```python
from build123d import *

# Parameters (mm, degrees)
BOSS_EXTRUDE1_DEPTH = 50
SKETCH2_W           = 15.285287044
SKETCH2_H           = 2
BOSS_EXTRUDE2_DEPTH = 10
FILLET1_R           = 2
SKETCH3_W           = 10
SKETCH3_H           = 26
SKETCH3_W_2         = 9.897545425
SKETCH3_H_2         = 19
CUT_EXTRUDE1_DEPTH  = 6
SKETCH4_W           = 2
SKETCH4_H           = 5
CUT_EXTRUDE2_DEPTH  = 31
FILLET2_R           = 4
FILLET3_R           = 2


with BuildPart() as part:
    # Sketch1 → Boss-Extrude1 (new body)
    with BuildSketch(Plane(origin=(0, 0, 0), x_dir=(1, 0, 0), z_dir=(0, 1, 0))):
        with BuildLine():
            Line((-5.276963181, 0), (34.723036819, 0))
            Line((34.723036819, 0), (34.723036819, 5))
            Line((34.723036819, 5), (24.723036819, 5))
            Line((24.723036819, 5), (24.723036819, 24))
            Line((24.723036819, 24), (22.365680341, 24))
            ThreePointArc((22.365680341, 24), (14.723036819, 14.1), (7.080393297, 24))
            Line((7.080393297, 24), (4.723036819, 24))
            Line((4.723036819, 24), (4.723036819, 5))
            Line((4.723036819, 5), (-5.276963181, 5))
            Line((-5.276963181, 5), (-5.276963181, 0))
        make_face()
    extrude(amount=BOSS_EXTRUDE1_DEPTH)

    # Sketch2 → Boss-Extrude2 (add)
    with BuildSketch(Plane(origin=(0, 0, -16), x_dir=(-1, 0, 0), z_dir=(0, 0, -1))):
        with Locations((-14.723036819, 49)):
            Rectangle(SKETCH2_W, SKETCH2_H)
        with Locations((-14.723036819, 1)):
            Rectangle(SKETCH2_W, SKETCH2_H)
    extrude(amount=-BOSS_EXTRUDE2_DEPTH)

    # Fillet1
    fillet1_edges = [part.edges().sort_by_distance(p)[0] for p in [
        (34.723036819, 50, -2.5),
        (34.723036819, 0, -2.5),
        (-5.276963181, 0, -2.5),
        (4.723036819, 25, -24),
        (24.723036819, 25, -24),
        (-5.276963181, 50, -2.5),
    ]]
    fillet(fillet1_edges, radius=FILLET1_R)

    # Sketch3 → Cut-Extrude1 (cut, through all)
    with BuildSketch(Plane(origin=(0, 0, -5), x_dir=(-1, 0, 0), z_dir=(0, 0, -1))):
        with BuildLine():
            Line((-0.723036819, 27.5), (0.776963181, 27.5))
            ThreePointArc((0.776963181, 27.5), (3.276963181, 25), (0.776963181, 22.5))
            Line((0.776963181, 22.5), (-0.723036819, 22.5))
            ThreePointArc((-0.723036819, 22.5), (-3.223036819, 25), (-0.723036819, 27.5))
        make_face()
        with BuildLine():
            Line((-30.223036819, 46.5), (-28.723036819, 46.5))
            ThreePointArc((-28.723036819, 46.5), (-26.223036819, 44), (-28.723036819, 41.5))
            Line((-28.723036819, 41.5), (-30.223036819, 41.5))
            ThreePointArc((-30.223036819, 41.5), (-32.723036819, 44), (-30.223036819, 46.5))
        make_face()
        with Locations((-29.723036819, 25)):
            Rectangle(SKETCH3_W, SKETCH3_H)
        with BuildLine():
            Line((-30.223036819, 8.5), (-28.723036819, 8.5))
            ThreePointArc((-28.723036819, 8.5), (-26.223036819, 6), (-28.723036819, 3.5))
            Line((-28.723036819, 3.5), (-30.223036819, 3.5))
            ThreePointArc((-30.223036819, 3.5), (-32.723036819, 6), (-30.223036819, 8.5))
        make_face()
        with Locations((0.328190468, 40.5)):
            Rectangle(SKETCH3_W_2, SKETCH3_H_2)
        with Locations((0.328190468, 9.5)):
            Rectangle(SKETCH3_W_2, SKETCH3_H_2)
    extrude(amount=-CUT_EXTRUDE1_DEPTH, mode=Mode.SUBTRACT)

    # Sketch4 → Cut-Extrude2 (cut, through all)
    with BuildSketch(Plane.ZY.offset(-4.723036819)):
        with Locations((-9.802694021, 42.5)):
            Rectangle(SKETCH4_W, SKETCH4_H)
        with Locations((-9.802694021, 7.5)):
            Rectangle(SKETCH4_W, SKETCH4_H)
    extrude(amount=-CUT_EXTRUDE2_DEPTH, mode=Mode.SUBTRACT)

    # Fillet2
    fillet2_edges = [part.edges().sort_by_distance(p)[0] for p in [
        (24.723036819, 42.5, -10.802694021),
        (4.723036819, 42.5, -10.802694021),
        (24.723036819, 7.5, -10.802694021),
        (4.723036819, 7.5, -10.802694021),
    ]]
    fillet(fillet2_edges, radius=FILLET2_R)

    # Fillet3
    fillet3_edges = [part.edges().sort_by_distance(p)[0] for p in [
        (34.723036819, 12, -2.5),
        (34.723036819, 38, -2.5),
        (-5.276963181, 31, -2.5),
        (-5.276963181, 19, -2.5),
    ]]
    fillet(fillet3_edges, radius=FILLET3_R)


solid = part.part
```
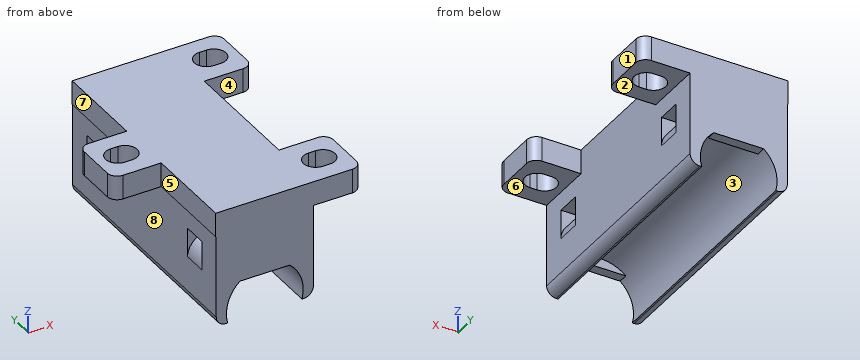
Verification items for the finished model (mm, model axes). Face numbers are marked on the shaded views. A direction names the side the tool comes from. Coordinates: 2 decimals unless noted, no trailing zeros. Write each loop counter-clockwise with the first axis right and the second up, starting at its lowest first coordinate (ties: lowest second). Pieces come first, ordered by that corner, then holes. Notation, with made-up numbers: M 7,57 L 28,57 A10 ccw 28,66 Z; hole C -12,75 d1. An arc over 180 degrees is marked long. One line per item, written item: value.
Item 1: Section check B-B, the plane y = 6. Record the boundary of the cut face in (x, z).
Check sheet entries:
outline: M 4.62,-5 L 4.72,-5 L 4.72,-8.8 L 24.72,-8.8 L 24.72,-5 L 26.22,-5 L 26.22,0 L 4.62,0 Z; M 4.72,-22 A2 ccw 6.72,-24 L 7.08,-24 A7.9 cw long 22.37,-24 L 22.72,-24 A2 ccw 24.72,-22 L 24.72,-14.8 A4 ccw 20.72,-10.8 L 8.72,-10.8 A4 ccw 4.72,-14.8 Z; M 32.72,-5 L 34.72,-5 L 34.72,0 L 32.72,0 Z
Item 2: Mould release check, pull along X, two halves, no side actions. Record for the marked faces 1, 2 and 3: pulls with the +X half, pulls with the -X half, needs draft (parallel to the pull), parting line crosses it, or undercut.
Check sheet entries:
face 1: pulls with the +X half
face 2: needs draft
face 3: undercut
Item 3: Access from +Z, -Z, +X, -X, +Y, -Y to the whole of each face (thin tool, end or side, straight path). Record for the marked faces 4, 5, 6, 7 and 8.
Check sheet entries:
face 4: +Z, -Z, +X
face 5: +Z, -Z, -X, -Y
face 6: -Z, +X, +Y, -Y
face 7: +Z, -Z, -X, +Y
face 8: -Z, -X, +Y, -Y
Item 4: Scan lines: line 1 along Y through (x, z) = (22, -9.5); line 2 along X through (y, z) = (34, -22); line 3 along X through (y, z) = (11, -16). Record each from-to range of solid material in increasing order.
Check sheet entries:
line 1: y = 0 to 5, 10 to 40, 45 to 50
line 2: x = 4.72 to 6.82, 22.62 to 24.72
line 3: x = 4.72 to 9.58, 19.86 to 24.72
Item 5: Section check D-D, the plane z = -18.25. Record the boundary of the cut face in (x, y), plus the area to 3 significant figures.
Check sheet entries:
outline: M 4.72,0 L 7.77,0 L 7.77,50 L 4.72,50 Z; M 21.68,0 L 24.72,0 L 24.72,50 L 21.68,50 Z
area: 305 mm^2
Item 6: Gauge pin test, flat ends, axial feed: pin 1 Ø4 at (x, y) = (15, 26.5) entering from -Z; pin 2 Ø3 at (x, y) = (0.5, 26.5) entering from -Z; pin 3 Ø0.8 at (x, z) = (-0.5, -1.5) entering from +Y. Record the tip position at first contact, or that the pin passes through.
Check sheet entries:
pin 1: stops at z = -14.44
pin 2: stops at z = -5
pin 3: stops at y = 31
Item 7: Section check A-A, the plane y = 25. Record the boundary of the cut face in (x, z).
Check sheet entries:
outline: M -5.28,-5 L -3.28,-5 L -3.28,0 L -5.28,0 Z; M 3.22,-5 L 4.72,-5 L 4.72,-22 A2 ccw 6.72,-24 L 7.08,-24 A7.9 cw long 22.37,-24 L 22.72,-24 A2 ccw 24.72,-22 L 24.72,0 L 3.22,0 Z
Item 8: Section check C-C, the plane x = 10.5. Record the boundary of the cut face in (y, z).
Check sheet entries:
outline: M 0,-16 L 2,-16 L 2,-15.32 L 48,-15.32 L 48,-16 L 50,-16 L 50,0 L 0,0 Z; hole M 5,-10.8 L 10,-10.8 L 10,-8.8 L 5,-8.8 Z; hole M 40,-10.8 L 45,-10.8 L 45,-8.8 L 40,-8.8 Z
